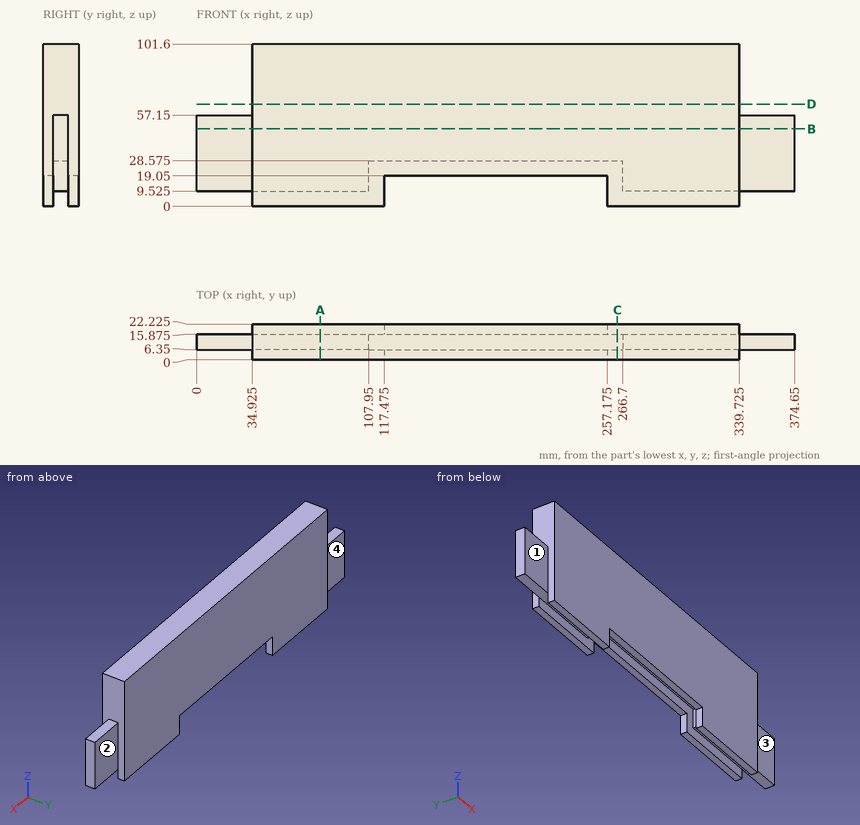
Input: dimensioned drawing with shaded views. Units: mm. Origin: part minimum x, y, z. A direction names the side the tool comes from. Give positions to 0.01 mm unless a question says otherwise; leave off trailing zeros. Loops run counter-clockwise (first coordinate to the right, second up) from the corner with the lowest first, then second, coordinate; pieces in that order, holes last. Notation, with made-up numbers: (79, 87) - (94, 87) arc R23 ccw to (94, 104) - close; hole circle Ø3 at (-17, -25). An arc over 180 degrees is marked (long way). Answer as CSV lines item,"result". Start each with the question number.
(1) Section query B-B (z = 48.5). Output: boundary loops of the cut face in (x, y) (3 decimals), and give its area (3 significant figures).
(2) Section query C-C (x = 263.5). Output: boundary loops of the cut face in (y, z) (3 decimals).
(3) Reachability of the marked faces 1, 2, 3 and 4 from +Z, -Z, +X, -X, +Y, -Y: full face, straight path, thin tool, end or side. Return the list, or none.
(4) Pin query (flat end, axial travel): P1, Ø1.5, axis at y = 19, z = 39, coming from the +X side (3 decimals); P2, Ø7.5, axis at x = 172.5, y = 12, coming from the -Z side (3 decimals); P3, Ø17.5, axis at x = 9, z = 21.5, coming from the -Y side; P4, Ø6, axis at y = 16, z = 20.5, coming from the -X side. Return the tip coordinate at first contact, or that it passes through.
(5) Section query A-A (x = 77.5). Output: boundary loops of the cut face in (y, z) (3 decimals), and give its area (3 significant figures).
(6) Section query D-D (z = 64). Output: boundary loops of the cut face in (x, y) (3 decimals).
(7) Ray query, line 1 along X through (y, z) = (21.5, 5) (3 decimals); line 2 along X through (y, z) = (13.25, 22); line 3 along Y through (x, z) = (63.5, 5) (3 decimals). Return the intervals inside material, ascending. Write a range as [from, to].
Worked answers:
1,outline,"(0, 6.35) - (34.925, 6.35) - (34.925, 0) - (339.725, 0) - (339.725, 6.35) - (374.65, 6.35) - (374.65, 15.875) - (339.725, 15.875) - (339.725, 22.225) - (34.925, 22.225) - (34.925, 15.875) - (0, 15.875) - close"
1,area,"7,440 mm^2"
2,outline,"(0, 0) - (6.35, 0) - (6.35, 28.575) - (15.875, 28.575) - (15.875, 0) - (22.225, 0) - (22.225, 101.6) - (0, 101.6) - close"
3,face 1,"+Z, -Z, -X, -Y"
3,face 2,"+Z, -Z, +X, +Y"
3,face 3,"+Z, -Z, +X, -Y"
3,face 4,"+Z, -Z, -X, +Y"
4,P1,"stops at x = 339.725"
4,P2,"stops at z = 28.575"
4,P3,"stops at y = 6.35"
4,P4,"stops at x = 0"
5,outline,"(0, 0) - (6.35, 0) - (6.35, 9.525) - (15.875, 9.525) - (15.875, 0) - (22.225, 0) - (22.225, 101.6) - (0, 101.6) - close"
5,area,"2,170 mm^2"
6,outline,"(34.925, 0) - (339.725, 0) - (339.725, 22.225) - (34.925, 22.225) - close"
7,line 1,"x = [34.925, 117.475], [257.175, 339.725]"
7,line 2,"x = [0, 107.95], [266.7, 374.65]"
7,line 3,"y = [0, 6.35], [15.875, 22.225]"
